from build123d import *

# Parameters (mm, degrees)
F2_R     = 4.7625
F3_DEPTH = 9.525
F4_R     = 1.5875
F5_DEPTH = 19.812


with BuildPart() as f1:
    # F0 (on Front) → F1 (revolve)
    with BuildSketch(Plane.XZ):
        with BuildLine():
            add(Edge.make_bspline(
                [(7.366, 25.4), (9.8036438765, 25.126718384), (14.9576453354, 23.9940702967), (23.5182465885, 21.2743691277), (25.4, 19.4404423237)],
                knots=[0, 0, 0, 0, 0.4619708182, 1, 1, 1, 1], degree=3))
            Line((7.366, 25.4), (7.366, 38.1))
            Line((7.366, 38.1), (0, 38.1))
            Line((0, 38.1), (0, 0))
            Line((0, 0), (2.1578229498, 0))
            Line((2.1578229498, 0), (7.5349872932, 8.6558889598))
            Line((7.5349872932, 8.6558889598), (25.4, 16.4627786726))
            Line((25.4, 16.4627786726), (25.4, 19.4404423237))
        make_face()
    revolve(axis=Axis((0, 0, 19.05), (0, 0, -1)))

    # F2 (on face) → F3 (cut)
    with BuildSketch(Plane.XY.offset(38.1)):
        Circle(F2_R)
    extrude(amount=-F3_DEPTH, mode=Mode.SUBTRACT)

    # F4 (on face) → F5 (cut)
    with BuildSketch(Plane(origin=(0, 0, 0), x_dir=(1, 0, 0), z_dir=(0, 0, -1))):
        Circle(F4_R)
    extrude(amount=-F5_DEPTH, mode=Mode.SUBTRACT)


solid = f1.part
Source: CAD feature listing. Evaluate the final solid. Frame: model axes, mm. A direction names the side the tool comes from. Round coordinates to 2 decimals unless told otherwise and drop trailing zeros. Loops run counter-clockwise (first coordinate to the right, second up) from the corner with the lowest first, then second, coordinate; pieces in that order, holes last. Notation, with made-up numbers: (81, -35) - (138, -35) arc R25 ccw to (138, -8) - close; hole circle Ø5 at (-4, 28). An arc over 180 degrees is marked (long way). Write item = value, one per line. Start each with the question number.
(1) Set-up query: faces 1 (the face through (0, 0, 19.812)), 2 (the face through (5, 0, 38.1)), 3 (the face through (3.399, 6.535, 31.839)). Return all of +Z, -Z, +X, -X, +Y, -Y with unobstructed straight access to the full face (end or side cutting, diameter ignored); none if empty.
(2) Section query A-A, the plane z = 13. Output: boundary loops of the cut face in (x, y) (1 decimal), plus the area to 3 significant figures.
(3) Pull-direction query (Y, two-part tool) for faces 4 (the face through (0, 0, 28.575)), 5 (the face through (-5.506, 24.796, 17.972)), 6 (the face through (0, -2, 0)); classes: +Y half, -Y half, draft (parallel to the pull), parting line (faces both ways), or undercut.
(4) Pin query (flat end, axial travel): pin 1 (6 mm diameter, centred on y = -4.5, z = 5, fed in from -X); pin 2 (4 mm diameter, centred on x = 0, y = 0, fed in from +Z) (3 decimals); pin 3 (10 mm diameter, centred on x = 0, z = 7, fed in from -Y); pin 4 (2.5 mm diameter, centred on x = -0.5, y = 0.5, fed in from -Z). Return the tip coordinate at first contact, or that it passes through.
(5) Ray query, line 1 along Y through (x, z) = (0, 34.5); line 2 along X through (y, z) = (0, 6); line 3 along Y through (x, z) = (-1, 3). Return the intervals inside material, ascending. Write a range as from..to.
Conclusion:
q1.face_1 = -Z
q1.face_2 = +Z, +X, -X, +Y, -Y
q1.face_3 = +Z
q2.outline = circle Ø35 at (0, 0); hole circle Ø3.2 at (0, 0)
q2.area = 952 mm2
q3.face_4 = undercut
q3.face_5 = parting line
q3.face_6 = draft
q4.pin_1 = -6.2
q4.pin_2 = 28.575
q4.pin_3 = -15.19
q4.pin_4 = 0
q5.line_1 = -7.37..-4.76, 4.76..7.37
q5.line_2 = -5.89..-1.59, 1.59..5.89
q5.line_3 = -3.9..-1.23, 1.23..3.9
